Geometry check sheet. Reference: the model listing, model coordinates, mm. Face numbers are marked on the shaded views. A direction names the side the tool comes from. Give positions to 0.01 mm unless a question says otherwise; leave off trailing zeros. Loops run counter-clockwise (first coordinate to the right, second up) from the corner with the lowest first, then second, coordinate; pieces in that order, holes last. Notation, with made-up numbers: (-23, -12.75) -> (-1, -12.75) arc R32 cw to (-1, 18.25) -> close; hole circle Ø7 at (72, -18.5). An arc over 180 degrees is marked (long way). Answer in a Markdown table with one row per item. Add a question column.
Autodesk Inventor part; units mm, degrees
ref_plane "YZ Plane" through (0, 0, 0) normal (1, 0, 0) x (0, 1, 0)
ref_plane "XZ Plane" through (0, 0, 0) normal (0, 1, 0) x (-1, 0, 0)
ref_plane "XY Plane" through (0, 0, 0) normal (0, 0, 1) x (1, 0, 0)
sketch "Sketch1" plane through (0, 0, 0) normal (0, 0, 1) x (1, 0, 0)
  circle A0 centre (0, 0) radius 50
  dimension "d0" = 100
extrude "Extrusion1" add sketch "Sketch1" along normal blind 12
sketch "Sketch2" plane through (0, 0, 0) normal (0, 0, -1) x (-1, 0, 0)
  circle A0 centre (0, 0) radius 15
  dimension "d3" = 30
extrude "Extrusion2" add sketch "Sketch2" along normal blind 12
chamfer "Chamfer1" distance 0.7 angle 45 1 edges at (-50, 0, 0)
chamfer "Chamfer2" distance 0.7 angle 45 1 edges at (-50, 0, 12)
sketch "Sketch9" plane through (0, 0, -12) normal (0, 0, -1) x (-1, 0, 0)
  circle A0 centre (0, 0) radius 6
  circle A1 centre (0, 0) radius 4
  dimension "d32" = 12
  dimension "d33" = 8
extrude "Extrusion9" add sketch "Sketch9" along normal blind 12
sketch "Sketch10" plane through (0, 0, 12) normal (0, 0, 1) x (1, 0, 0)
  circle A0 centre (0, 0) radius 49.3
  line L0 (-46.9792, -14.9479) -> (-32.0415, 0)
  line L1 (-32.0415, 0) -> (-34.8474, 0)
  line L2 (-46.9792, 14.9479) -> (-32.0415, 0)
  line L3 (-46.9792, -14.9479) -> (-50.9309, -18.8996)
  line L4 (-46.9792, -14.9479) -> (-41.3907, -14.9479) construction
  line L5 (-46.9792, 14.9479) -> (-50.9309, 18.8996)
  arc A1 (-50.9309, 18.8996) -> (-50.9309, -18.8996) centre (-5.1445, 0) ccw
  arc A2 (-46.9792, 14.9479) -> (-46.9792, -14.9479) centre (0, 0) ccw
  line L6 (-17.4257, 0) -> (-43.6281, 26.2024)
  line L7 (-17.4257, 0) -> (19.6301, 0) construction
  line L8 (-12.476, 4.9497) -> (-38.6784, 31.1522)
  line L9 (-17.4257, 0) -> (-12.476, 4.9497)
  arc A3 (-38.4198, 30.8935) -> (-42.4668, 25.0411) centre (0, 0) ccw
  arc A4 (-38.6784, 31.1522) -> (-43.6281, 26.2024) centre (-36.0468, 23.5708) ccw
  dimension "d36" = 135
  dimension "d39" = 135
extrude "Extrusion10" cut sketch "Sketch10" against normal blind 8 contours L3 A1 L5 A0 | A0 L2 L0
sketch "Sketch11" plane through (0, 0, 12) normal (0, 0, 1) x (1, 0, 0)
  line L0 (-46.9792, 14.9479) -> (-32.0415, 0)
  line L1 (-39.5104, 7.474) -> (-34.5589, 12.422)
  line L2 (-22.1379, 0.0075) -> (-44.1228, 21.9924)
  circle A0 centre (0, 0) radius 49.3
  line L3 (-34.5589, 12.422) -> (-29.6092, 17.3718)
  line L4 (-34.5589, 12.422) -> (-27.5589, 12.422) construction
  line L5 (-32.0841, 14.8969) -> (-29.6092, 12.422)
  line L6 (-17.1946, 4.9507) -> (-39.1796, 26.9357)
  line L7 (-22.1379, 0.0075) -> (-17.1946, 4.9507)
  line L8 (-39.1796, 26.9357) -> (-40.4406, 28.1966)
  line L9 (-44.1228, 21.9924) -> (-46.2441, 24.1138)
  line L10 (-40.4406, 28.1966) -> (-42.3953, 30.4724)
  arc A1 (-42.3953, 30.4724) -> (-46.289, 24.1586) centre (-36.8863, 22.7176) ccw
  arc A2 (-46.9792, -14.9479) -> (-46.9792, 14.9479) centre (0, 0) ccw
  point P0 (-34.5557, 12.4253)
  point P1 (-29.6124, 17.3685)
  dimension "d42" = 7
  dimension "d43" = 7
  dimension "d45" = 3
  dimension "d46" = 3
extrude "Extrusion11" cut sketch "Sketch11" against normal blind 8 contours A0 L8 L6 L3 L2
sketch "Sketch12" plane through (-46.9792, 14.9479, 4) normal (-0.7073, -0.7069, 0) x (0, 0, 1)
  circle A0 centre (3.8047, -3.4144) radius 1.5
  point P0 (-4, -43.7814)
  dimension "d49" = 3
extrude "Extrusion12" cut sketch "Sketch12" against normal blind 8
properties part number "FlyCutter"
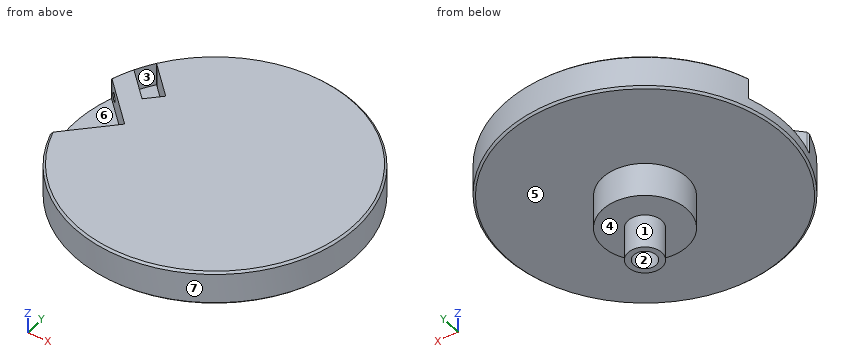
1. Release check for a two-part mould opening along X. For the marked faces 1, 2, 3 and 4 record: released by +X, released by -X, zero draft, split by the parting line, or undercut.
2. Sectioned sample at D-D (z = -2). Enter the section's corners in (x, y).
3. Sectioned sample at A-A (x = 0). Enter the section's corners in (y, z), plus the area to 3 significant figures.
4. Sectioned sample at C-C (z = 8). Enter the section's corners in (x, y), plus the area to 3 significant figures.
5. Access from +Z, -Z, +X, -X, +Y, -Y to the whole of each face (thin tool, end or side, straight path). Record for the marked faces 5, 6 and 7.
6. Gauge pin test, flat ends, axial feed: pin 1 Ø1.5 at (x, y) = (19, -23.5) entering from -Z; pin 2 Ø1.5 at (x, z) = (-27, 0) entering from +Y; pin 3 Ø12 at (y, z) = (31, 0.5) entering from +X. Record the tip position at first contact, or that the pin passes through.
7. Material ranges on L1, parallel to Y at x = 0, z = -20.75; L2, parallel to Y at x = -36.5, z = 8; L3, parallel to Z at x = 13.5, y = 42, recorded low to high. Write a range as from..to.
8. Sectioned sample at B-B (z = -15.5). Enter the section's corners in (x, y).
Response:
| question | item | result |
|---|---|---|
| 1 | face 1 | split by the parting line |
| 1 | face 2 | undercut |
| 1 | face 3 | undercut |
| 1 | face 4 | zero draft |
| 2 | outline | circle Ø30 at (0, 0) |
| 3 | outline | (-50, 0.7) -> (-49.3, 0) -> (-15, 0) -> (-15, -12) -> (-6, -12) -> (-6, -24) -> (-4, -24) -> (-4, -12) -> (4, -12) -> (4, -24) -> (6, -24) -> (6, -12) -> (15, -12) -> (15, 0) -> (49.3, 0) -> (50, 0.7) -> (50, 11.3) -> (49.3, 12) -> (-49.3, 12) -> (-50, 11.3) -> close |
| 3 | area | 1,610 mm2 |
| 4 | outline | (-47.54, -15.5) arc R50 ccw (long way) to (-47.54, 15.5) -> (-46.98, 14.95) -> (-45.62, 13.58) -> (-40.66, 18.53) -> (-44.12, 21.99) arc R49.3 cw to (-40.44, 28.2) -> (-39.18, 26.94) -> (-29.61, 17.37) -> (-34.56, 12.43) -> (-38.56, 16.43) -> (-43.51, 11.48) -> (-32.04, 0) -> (-46.98, -14.95) -> close |
| 4 | area | 7,440 mm2 |
| 5 | face 5 | -Z |
| 5 | face 6 | +Z, -X |
| 5 | face 7 | +Z, -Z |
| 6 | pin 1 | stops at z = 0 |
| 6 | pin 2 | stops at y = 42.26 |
| 6 | pin 3 | stops at x = 43.3 |
| 7 | L1 | y = -6..-4, 4..6 |
| 7 | L2 | y = -34.17..-4.46, 4.46..14.37, 24.26..34.17 |
| 7 | L3 | z = 0..12 |
| 8 | outline | circle Ø12 at (0, 0); hole circle Ø8 at (0, 0) |
